Design review of the part built by this model. Coordinates are the model's own, in mm. Coordinates: 2 decimals unless noted, no trailing zeros. Loops run counter-clockwise (first coordinate to the right, second up) from the corner with the lowest first, then second, coordinate; pieces in that order, holes last. Notation, with made-up numbers: M 81.5,-7 L 103.5,-7 A25 ccw 103.5,23 Z; hole C -8.5,73 d4. An arc over 180 degrees is marked long. Write item = value, one per line. Start each with the question number.
from build123d import *

# Parameters (mm, degrees)
SKETCH1_W           = 20.32
SKETCH1_H           = 81.316938585
BOSS_EXTRUDE1_DEPTH = 10.16


with BuildPart() as part:
    # Sketch1 → Boss-Extrude1 (new body)
    with BuildSketch(Plane.XY):
        with BuildLine():
            Line((-444.5, 10.16), (-321.2, 10.16))
            Line((-321.2, 10.16), (-321.2, 0))
            Line((-321.2, 0), (-245, 0))
            Line((-245, 0), (-245, 10.16))
            Line((-245, 10.16), (-38.1, 10.16))
            Line((-38.1, 10.16), (-38.1, 0))
            Line((-38.1, 0), (38.1, 0))
            Line((38.1, 0), (38.1, 10.16))
            Line((38.1, 10.16), (245, 10.16))
            Line((245, 10.16), (245, 0))
            Line((245, 0), (321.2, 0))
            Line((321.2, 0), (321.2, 10.16))
            Line((321.2, 10.16), (444.500003861, 10.16))
            add(Edge.make_bspline(
                [(444.500003861, 10.16), (519.890985801, 10.806562601), (520.046520423, 86.2)],
                knots=[4.720964914, 4.720964914, 4.720964914, 6.281122341, 6.281122341, 6.281122341], degree=2, weights=[1, 0.710858178, 1]))
            Line((520.046520423, 86.2), (520.070316185, 435.449980504))
            Line((520.070316185, 435.449980504), (205.706405146, 435.61))
            Line((205.706405146, 435.61), (205.558012439, 425.45))
            Line((205.558012439, 425.45), (123.444, 425.45))
            Line((123.444, 425.45), (123.444, 435.61))
            Line((123.444, 435.61), (41.148, 435.61))
            Line((41.148, 435.61), (41.148, 425.45))
            Line((41.148, 425.45), (-41.148, 425.45))
            Line((-41.148, 425.45), (-41.148, 435.61))
            Line((-41.148, 435.61), (-123.444, 435.61))
            Line((-123.444, 435.61), (-123.444, 425.45))
            Line((-123.444, 425.45), (-205.74, 425.45))
            Line((-205.74, 425.45), (-205.74, 388.35))
            Line((-205.74, 388.35), (-230.359692718, 388.35))
            Line((-230.359692718, 388.35), (-230.359692718, 498.154928973))
            Line((-230.359692718, 498.154928973), (-530.359692718, 498.154928973))
            Line((-530.359692718, 498.154928973), (-530.359692718, 469.654928973))
            Line((-530.359692718, 469.654928973), (-520.360110714, 469.746360594))
            Line((-520.360110714, 469.746360594), (-520.360110714, 435.61))
            Line((-520.360110714, 435.61), (-520.7, 86.36))
            ThreePointArc((-520.7, 86.36), (-498.381536726, 32.478463274), (-444.5, 10.16))
        make_face()
        with Locations((206.375268781, 132.135407878)):
            Rectangle(SKETCH1_W, SKETCH1_H, mode=Mode.SUBTRACT)
        with Locations((206.375268781, 294.769285048)):
            Rectangle(SKETCH1_W, SKETCH1_H, mode=Mode.SUBTRACT)
        with Locations((-206.375268781, 132.135407878)):
            Rectangle(SKETCH1_W, SKETCH1_H, mode=Mode.SUBTRACT)
        with Locations((-206.375268781, 294.769285048)):
            Rectangle(SKETCH1_W, SKETCH1_H, mode=Mode.SUBTRACT)
    extrude(amount=BOSS_EXTRUDE1_DEPTH)


solid = part.part
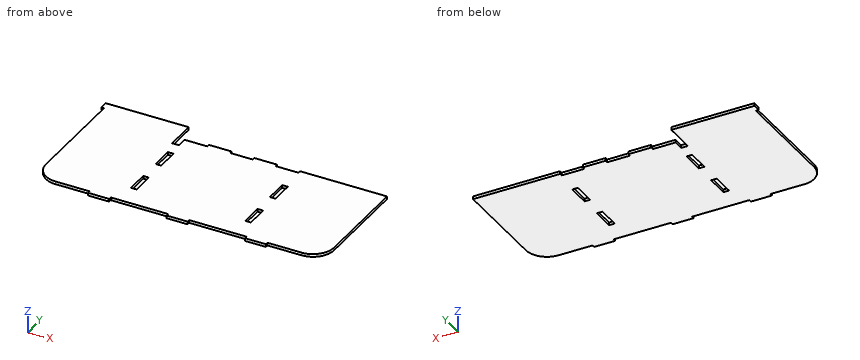
Q1. Add section C-C on z = 5.75. Give the number of separate pieces and of enclosed holes in the cut face, plus the area to 3 significant figures.
Q2. Add section D-D on x = -402. State the section outline as (y, z) points, plus the area to 3 significant figures.
Q3. To check wall thickness, follow line 1 (Y direction, x = 215, z = 1.75); line 2 (X direction, y = 266.5, z = 8.25); line 3 (X direction, y = 426, z = 4.75). State the ranges of each line that lie inside material, in increasing order. Write a range as from..to.
Q4. Add section B-B on x = -58. State the section outline as (y, z) points, plus the area to 3 significant figures.
Q5. Clearance check with flat-ended pins moving along their axes: P1, Ø1.5, axis at y = 155, z = 1.5, coming from the -X side; P2, Ø5, axis at y = 6, z = 7, coming from the -X side; P3, Ø5, axis at y = 289, z = 6.5, coming from the -X side. State where each tip first meets the part, or that it passes through.
Q6. Add section A-A on y = 299.5. State the section outline as (x, z) points.
Values follow:
q1.separate_pieces = 1
q1.enclosed_holes = 4
q1.area = 451,000 mm2
q2.outline = M 10.16,0 L 498.15,0 L 498.15,10.16 L 10.16,10.16 Z
q2.area = 4,960 mm2
q3.line_1 = 10.16..91.48, 172.79..254.11, 335.43..435.61
q3.line_2 = -520.52..-216.54, -196.22..196.22, 216.54..520.06
q3.line_3 = -520.37..-230.36, -123.44..-41.15, 41.15..123.44, 205.57..520.07
q4.outline = M 10.16,0 L 435.61,0 L 435.61,10.16 L 10.16,10.16 Z
q4.area = 4,320 mm2
q5.P1 = -520.63
q5.P2 = -321.2
q5.P3 = -520.51
q6.outline = M -520.49,0 L -216.54,0 L -216.54,10.16 L -520.49,10.16 Z; M -196.22,0 L 196.22,0 L 196.22,10.16 L -196.22,10.16 Z; M 216.54,0 L 520.06,0 L 520.06,10.16 L 216.54,10.16 Z
